Geometry: see drawing. Coordinates: mm, zero at the bounding-box minimum. Round coordinates to 2 decimals unless told otherwise and drop trailing zeros. Order: outer loops, then holes, each group sorted by start corner. A loop starts at its lowest first (then second) coordinate and runs counter-clockwise, first axis right, second up. Notation, with made-up numbers: (20.5, -20) -> (60.5, -20) arc R10 cw to (60.5, -12) -> close; hole circle Ø1 at (-20, 81.5). An arc over 180 degrees is marked (long way). Use a Markdown table: item, result.
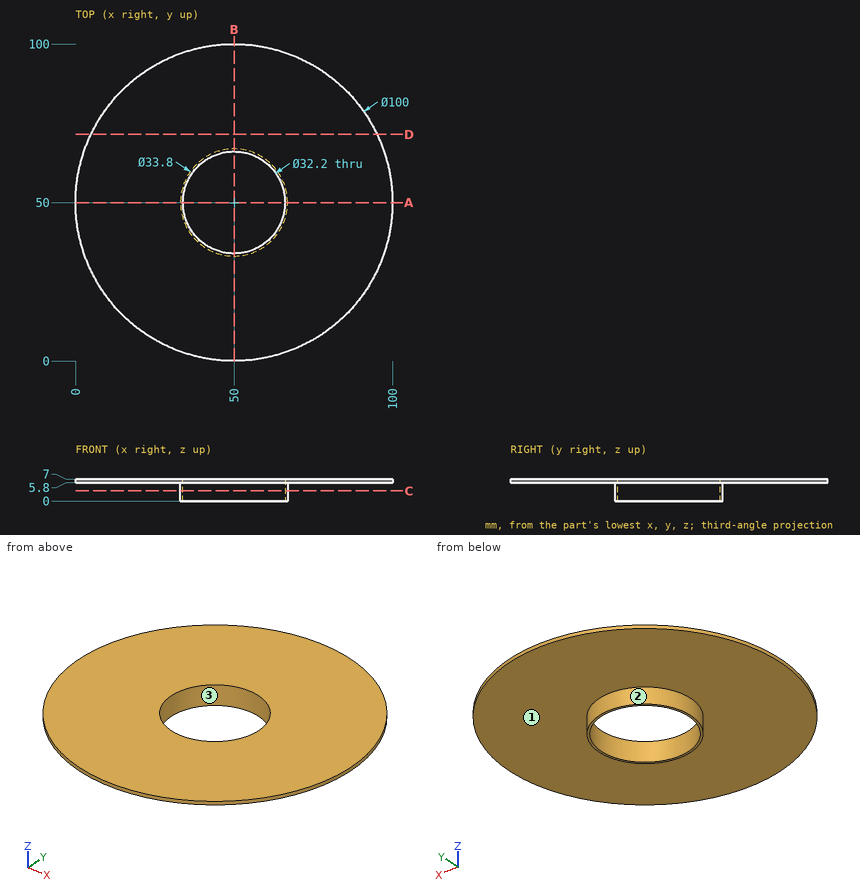
1) Contact query for flat-ended pins moving along their axis: P1, Ø1.5, axis at y = 44, z = 5.5, coming from the +X side; P2, Ø3, axis at x = 30.5, z = 6, coming from the -Y side. Output: stop coordinate, or through.
Answer key:
| item | result |
|---|---|
| P1 | stops at x = 99.72 |
| P2 | stops at y = 3.35 |
2) Draft query along X for the marked faces 1, 2 and 3. Return one class per face: released by +X, released by -X, zero draft, split by the parting line, or undercut.
Answer key:
| item | result |
|---|---|
| face 1 | zero draft |
| face 2 | split by the parting line |
| face 3 | undercut |
3) Cut plane D-D on y = 71.5. Return loops of the section in (x, z), and give its area (3 significant figures).
Answer key:
| item | result |
|---|---|
| outline | (4.86, 5.8) -> (95.14, 5.8) -> (95.14, 7) -> (4.86, 7) -> close |
| area | 108 mm^2 |
4) Cut plane A-A on y = 50. Return loops of the section in (x, z), and give its area (3 significant figures).
Answer key:
| item | result |
|---|---|
| outline | (0, 5.8) -> (33.1, 5.8) -> (33.1, 0) -> (33.9, 0) -> (33.9, 7) -> (0, 7) -> close; (66.1, 0) -> (66.9, 0) -> (66.9, 5.8) -> (100, 5.8) -> (100, 7) -> (66.1, 7) -> close |
| area | 90.6 mm^2 |
5) Ray query, probe 1 along Y at (x, z) = (50, 5.5); probe 2 along Z at (x, y) = (81.5, 41.5). Return the intervals inside material, ascending.
Answer key:
| item | result |
|---|---|
| probe 1 | y = 33.1 to 33.9, 66.1 to 66.9 |
| probe 2 | z = 5.8 to 7 |
6) Cut plane C-C on z = 3.25. Return loops of the section in (x, y).
Answer key:
| item | result |
|---|---|
| outline | circle Ø33.8 at (50, 50); hole circle Ø32.2 at (50, 50) |
